Autodesk Inventor part; units mm, degrees
ref_plane "YZ Plane" through (0, 0, 0) normal (1, 0, 0) x (0, 1, 0)
ref_plane "XZ Plane" through (0, 0, 0) normal (0, 1, 0) x (-1, 0, 0)
ref_plane "XY Plane" through (0, 0, 0) normal (0, 0, 1) x (1, 0, 0)
sketch "Sketch1" plane through (0, 0, 0) normal (0, 1, 0) x (-1, 0, 0)
  line L0 (8.8257, 8.4823) -> (-21.1743, 8.4823)
  line L1 (-21.1743, 8.4823) -> (-21.1743, -13.5177)
  line L2 (-21.1743, -13.5177) -> (8.8257, -13.5177)
  line L3 (8.8257, -13.5177) -> (8.8257, 8.4823)
  point P0 (0, 0)
  dimension "d0" = 30
  dimension "d1" = 22
extrude "Extrusion1" add sketch "Sketch1" along normal blind 6
fillet "Fillet1" radius 4 4 edges at (21.1743, 3, 8.4823) (21.1743, 3, -13.5177) (-8.8257, 3, -13.5177) (-8.8257, 3, 8.4823)
sketch "Sketch3" plane through (21.1743, 0, 4.4823) normal (1, 0, 0) x (0, 0, -1)
  line L0 (0, 0) -> (14, 0)
  line L1 (0, 6) -> (14, 6)
  line L2 (14, 6) -> (14, 0)
  line L3 (0, 0) -> (0, 6)
  line L4 (0, 0) -> (0, 6)
  line L5 (0, 6) -> (14, 6)
  arc A0 (9.6269, 0) -> (4.3731, 0) centre (7, -1.5) ccw
  dimension "d35" = 7
  dimension "d37" = 6.05
  dimension "d40" = 1.5
  dimension "d41" = 14
sketch "Sketch4" plane through (-8.8257, 0, -9.5177) normal (-1, 0, 0) x (0, 0, 1)
  line L0 (0, 0) -> (14, 0)
  line L1 (0, 0) -> (14, 0)
  line L2 (0, 6) -> (0, 0)
  line L3 (0, 0) -> (0, 6)
  line L4 (14, 6) -> (0, 6)
  line L5 (0, 6) -> (14, 6)
  line L6 (14, 0) -> (14, 6)
  line L7 (14, 6) -> (14, 0)
  arc A0 (9.093, 0) -> (4.907, 0) centre (7, -1.5) ccw
  dimension "d31" = 7
  dimension "d32" = 5.15
  dimension "d42" = 14
  dimension "d43" = 1.5
extrude "Extrusion5" cut sketch "Sketch4" against normal blind 15 contours A0 L0
extrude "Extrusion6" cut sketch "Sketch3" against normal blind 15 contours A0 L0
sketch "Szkic5" plane through (0, 0, 0) normal (0, -1, 0) x (1, 0, 0)
  line L0 (6.1743, 0.1092) -> (21.1743, 0.1092)
  line L1 (21.1743, 4.4823) -> (21.1743, 0.1092)
  arc A0 (21.1743, 4.4823) -> (17.1743, 8.4823) centre (17.1743, 4.4823) ccw
  line L2 (-4.8257, 8.4823) -> (17.1743, 8.4823)
  arc A1 (-4.8257, 8.4823) -> (-8.8257, 4.4823) centre (-4.8257, 4.4823) ccw
  line L3 (-8.8257, -0.4247) -> (-8.8257, 4.4823)
  line L4 (-8.8257, -0.4247) -> (6.1743, -0.4247)
  line L5 (6.1743, -0.4247) -> (6.1743, 0.1092)
  line L6 (21.1743, -5.1446) -> (6.1743, -5.1446)
  line L7 (6.1743, -5.1446) -> (6.1743, -4.6107)
  line L8 (6.1743, -4.6107) -> (-8.8257, -4.6107)
  line L9 (-8.8257, -9.5177) -> (-8.8257, -4.6107)
  arc A2 (-8.8257, -9.5177) -> (-4.8257, -13.5177) centre (-4.8257, -9.5177) ccw
  line L10 (17.1743, -13.5177) -> (-4.8257, -13.5177)
  arc A3 (17.1743, -13.5177) -> (21.1743, -9.5177) centre (17.1743, -9.5177) ccw
  line L11 (21.1743, -5.1446) -> (21.1743, -9.5177)
  point P0 (0, 0)
  point P1 (14.1743, 4.2958)
  point P2 (-1.8257, 4.0288)
  point P3 (14.1743, -9.3311)
  point P4 (-1.8257, -9.0642)
  dimension "d44" = 7
  dimension "d45" = 7
  dimension "d46" = 15
  dimension "d47" = 15
  dimension "d48" = 7
  dimension "d49" = 7
  dimension "d50" = 4.4535
  dimension "d51" = 4.4535
  dimension "d52" = 4.1866
  dimension "d53" = 4.1866
  dimension "d61" = 8.3731
  dimension "d62" = 8.907
hole "Otwór2" at (14.1743, 0, 4.2958) at (-1.8257, 0, 4.0288) at (14.1743, 0, -9.3311) at (-1.8257, 0, -9.0642) direction (0, 1, 0) diameter 3.2 end through all
properties part number "3DP_ABS_Z_Axis_Screw_Coupler"
Input: part model. Units: mm. Frame: model coordinates. A direction names the side the tool comes from. Give positions to 0.01 mm unless a question says otherwise; leave off trailing zeros. Order: outer loops, then holes, each group sorted by start corner. A loop starts at its lowest first (then second) coordinate and runs counter-clockwise, first axis right, second up. Notation, with made-up numbers: M 24,5.25 L 70,5.25 A24 cw 70,37.25 Z; hole C -39.5,-7.5 d1. An arc over 180 degrees is marked long. One line per question, with ' | ' between items. Start each with the question number.
1. Material intervals for probe 1 along Z at (x, y) = (-2.75, 4); probe 2 along Z at (x, y) = (-1, 3.25); probe 3 along X at (y, z) = (3, -8), sorted ascending. Write a range as [from, to].
2. Section query A-A (y = 0.5). Return the cut outline in (x, z).
3. Access query for faces 1 (the face through (6.174, 1.22, -2.31)), 2 (the face through (13.093, 3.042, 5.475)). Directions: +Z, -Z, +X, -X, +Y, -Y. A direction counts if a zero-diameter tool reaches every point of the face in a straight line with its end or side. Return the directions, or none.
4. Section query C-C (x = 15). Return the cut outline in (y, z) (3 decimals).
5. Section query D-D (y = 4.25). Return the cut outline in (x, z), and give its area (3 significant figures).
6. Pull-direction query (X, two-part tool) for faces 3 (the face through (-3.412, 3.042, -8.856)), 4 (the face through (19.971, 3.042, 7.342)), 5 (the face through (6, 0, 4)); classes: released by +X, released by -X, zero draft, split by the parting line, or undercut.
7. Section query B-B (x = 1.25). Return the cut outline in (y, z) (3 decimals).
8. First-contact query: pin 1 Ø3 at (x, z) = (14.17, -9.33) entering from +Y. Flat tip, straight axial feed; report the tip coordinate or a pass-through.
Here are the results:
1) probe 1: [-13.52, -10.37], [-7.76, 2.72], [5.33, 8.48] | probe 2: [-13.52, -10.43], [-7.69, 2.66], [5.4, 8.48] | probe 3: [-8.83, -3.02], [-0.63, 13.29], [15.06, 21.17]
2) outline: M -8.83,-9.52 A4 ccw -4.83,-13.52 L 17.17,-13.52 A4 ccw 21.17,-9.52 L 21.17,-4.79 L 6.17,-4.79 L 6.17,-4.14 L -8.83,-4.14 Z; M -8.83,-0.9 L 6.17,-0.9 L 6.17,-0.25 L 21.17,-0.25 L 21.17,4.48 A4 ccw 17.17,8.48 L -4.83,8.48 A4 ccw -8.83,4.48 Z; hole C -1.83,-9.06 d3.2; hole C -1.83,4.03 d3.2; hole C 14.17,-9.33 d3.2; hole C 14.17,4.3 d3.2
3) face 1: +X, -Y | face 2: +Y, -Y
4) outline: M 0,-13.518 L 6,-13.518 L 6,-10.702 L 0,-10.702 Z; M 0,-7.961 L 6,-7.961 L 6,2.925 L 0,2.925 L 0,0.109 A3.025 cw 0,-5.145 Z; M 0,5.666 L 6,5.666 L 6,8.482 L 0,8.482 Z
5) outline: M -8.83,-9.52 A4 ccw -4.83,-13.52 L 17.17,-13.52 A4 ccw 21.17,-9.52 L 21.17,4.48 A4 ccw 17.17,8.48 L -4.83,8.48 A4 ccw -8.83,4.48 Z; hole C -1.83,-9.06 d3.2; hole C -1.83,4.03 d3.2; hole C 14.17,-9.33 d3.2; hole C 14.17,4.3 d3.2 | area: 614 mm²
6) face 3: undercut | face 4: released by +X | face 5: zero draft
7) outline: M 0,-13.518 L 6,-13.518 L 6,8.482 L 0,8.482 L 0,-0.425 A2.575 cw 0,-4.611 Z
8) pin 1: through
